For this review, take the finished solid that the model builds, in its own axes (mm). A direction names the side the tool comes from. Coordinates: 2 decimals unless noted, no trailing zeros. Order: outer loops, then holes, each group sorted by start corner. A loop starts at its lowest first (then second) coordinate and runs counter-clockwise, first axis right, second up.
from build123d import *

# Parameters (mm, degrees)
F0_R     = 1.75
F0_R_2   = 15
F1_DEPTH = 4


with BuildPart() as f1:
    # F0 (on Top) → F1 (new body)
    with BuildSketch(Plane.XY):
        Polygon((23.931458, 9.5), (23.931458, 0), (35.75, 0), (35.75, 16), (54.25, 16), (54.25, 0), (66.068542, 0), (66.068542, 9.5), (80.900239, 23.931458), (90.006756, 23.931458), (90.006756, 35.75), (74.006756, 35.75), (74.006756, 54.25), (90.006756, 54.25), (90.006756, 66.068542), (80.900239, 66.068542), (66.068542, 80.5), (66.068542, 90), (54.25, 90), (54.25, 74), (35.75, 74), (35.75, 90), (23.931458, 90), (23.931458, 80.5), (9.5, 66.068542), (0.006756, 66.068542), (0.006756, 54.25), (16.006756, 54.25), (16.006756, 35.75), (0.006756, 35.75), (0.006756, 23.931458), (9.5, 23.931458), align=None)
        with Locations((28.931458, 8)):
            Circle(F0_R, mode=Mode.SUBTRACT)
        with Locations((8.006756, 28.931458)):
            Circle(F0_R, mode=Mode.SUBTRACT)
        with Locations((45, 23.433243)):
            Circle(F0_R, mode=Mode.SUBTRACT)
        with Locations((61.068542, 8)):
            Circle(F0_R, mode=Mode.SUBTRACT)
        with Locations((82.006757, 28.931458)):
            Circle(F0_R, mode=Mode.SUBTRACT)
        with Locations((8, 61.068542)):
            Circle(F0_R, mode=Mode.SUBTRACT)
        with Locations((23.433243, 45)):
            Circle(F0_R, mode=Mode.SUBTRACT)
        with Locations((45, 45)):
            Circle(F0_R_2, mode=Mode.SUBTRACT)
        with Locations((45, 66.566757)):
            Circle(F0_R, mode=Mode.SUBTRACT)
        with Locations((28.931458, 82)):
            Circle(F0_R, mode=Mode.SUBTRACT)
        with Locations((66.566757, 45)):
            Circle(F0_R, mode=Mode.SUBTRACT)
        with Locations((82.006756, 61.068542)):
            Circle(F0_R, mode=Mode.SUBTRACT)
        with Locations((61.068542, 82.006756)):
            Circle(F0_R, mode=Mode.SUBTRACT)
    extrude(amount=F1_DEPTH)


solid = f1.part
1. Machinability: for faces 4 (the face through (66.069, 5, 2)), 5 (the face through (23.931, 5, 2)), 6 (the face through (74.007, 45, 2)), 7 (the face through (45, 16, 2)), 8 (the face through (16.007, 45, 2)), which of the approach directions +Z, -Z, +X, -X, +Y, -Y give a long, thin tool a straight path to every point of the face, cutting with its end or side? Answer none if there is none.
Answer below:
face 4: +Z, -Z, +X, -Y
face 5: +Z, -Z, -X, -Y
face 6: +Z, -Z, +X
face 7: +Z, -Z, -Y
face 8: +Z, -Z, -X
2. Take a section at D-D, the plane x = 56. Give the boundary of the cut face in (y, z), plus the area to 3 significant figures.
Answer below:
outline: (0, 0) - (34.8, 0) - (34.8, 4) - (0, 4) - close; (55.2, 0) - (90, 0) - (90, 4) - (55.2, 4) - close
area: 278 mm2
3. Take a section at A-A, the plane x = 45. Give the boundary of the cut face in (y, z).
Answer below:
outline: (16, 0) - (21.68, 0) - (21.68, 4) - (16, 4) - close; (25.18, 0) - (30, 0) - (30, 4) - (25.18, 4) - close; (60, 0) - (64.82, 0) - (64.82, 4) - (60, 4) - close; (68.32, 0) - (74, 0) - (74, 4) - (68.32, 4) - close
4. Clearance check with flat-ended pins moving along their axes: pin 1 Ø1.2 at (x, z) = (6.5, 2.5) entering from +Y; pin 2 Ø3 at (x, y) = (82.01, 28.93) entering from -Z; pin 3 Ø2 at (y, z) = (43.5, 2) entering from +X; pin 4 Ø1.2 at (x, z) = (78, 1.5) entering from +Y. State where each tip first meets the part, or that it passes through.
Answer below:
pin 1: stops at y = 66.07
pin 2: passes through
pin 3: stops at x = 74.01
pin 4: stops at y = 69.47
5. The part is to be moulded in two halves that separate along Y. For faces 1 (the face through (5, 23.931, 2)), 2 (the face through (86, 66.069, 2)), 3 (the face through (83.676, 29.457, 1.972)), say which applies: +Y half, -Y half, draft (parallel to the pull), parting line (faces both ways), or undercut.
Answer below:
face 1: -Y half
face 2: +Y half
face 3: undercut
6. Take a section at C-C, the plane y = 32. Give the boundary of the cut face in (x, z), plus the area to 3 significant figures.
Answer below:
outline: (0.01, 0) - (37.52, 0) - (37.52, 4) - (0.01, 4) - close; (52.48, 0) - (90.01, 0) - (90.01, 4) - (52.48, 4) - close
area: 300 mm2
7. To check wall thickness, follow L1, parallel to X at y = 82, z = 2.4; L2, parallel to Y at x = 61, z = 0.2; L3, parallel to Y at x = 84.5, z = 2.9. State the ranges of each line that lie inside material, in increasing order.
Answer below:
L1: x = 23.93 to 27.18, 30.68 to 35.75, 54.25 to 59.32, 62.82 to 66.07
L2: y = 0 to 6.25, 9.75 to 80.26, 83.76 to 90
L3: y = 23.93 to 35.75, 54.25 to 66.07
8. Take a section at B-B, the plane y = 45. Give the boundary of the cut face in (x, z), plus the area to 3 significant figures.
Answer below:
outline: (16.01, 0) - (21.68, 0) - (21.68, 4) - (16.01, 4) - close; (25.18, 0) - (30, 0) - (30, 4) - (25.18, 4) - close; (60, 0) - (64.82, 0) - (64.82, 4) - (60, 4) - close; (68.32, 0) - (74.01, 0) - (74.01, 4) - (68.32, 4) - close
area: 84.0 mm2
